For this review, take the finished solid that the model builds, in its own axes (mm). Face numbers are marked on the shaded views. A direction names the side the tool comes from. Round coordinates to 2 decimals unless told otherwise and drop trailing zeros. Loops run counter-clockwise (first coordinate to the right, second up) from the corner with the lowest first, then second, coordinate; pieces in that order, holes last.
1. To check wall thickness, follow line 1 along X through (y, z) = (-23, -36); line 2 along Y through (x, z) = (-10.5, -35); line 3 along Z through (x, y) = (-66, -9.5). State the ranges of each line that lie inside material, in increasing order.
2. Tool access review of the marked faces 5, 6 and 7: name each direction out of +Z, -Z, +X, -X, +Y, -Y from which nothing blocks a thin tool from reaching the whole face with its end or side.
3. Consider section B-B on x = 68. State the section outline as (y, z) points.
4. Clearance check with flat-ended pins moving along their axes: pin 1 Ø10 at (x, z) = (22, -87) entering from +Y; pin 2 Ø8 at (x, y) = (45, -37.5) entering from +Z; pin 3 Ø2 at (x, z) = (12, -44) entering from -Y. State where each tip first meets the part, or that it passes through.
5. Consider section D-D on x = 30. State the section outline as (y, z) points, then the cut area to 3 significant figures.
6. Consider section C-C on y = -22. State how many separate pieces and enclosed holes the cut face has, then the cut area to 3 significant figures.
7. Draft analysis for pull direction Z (two halves, no side actions). For the marked faces 1, 2, 3 and 4, state which applies: released by +Z, released by -Z, zero draft, split by the parting line, or undercut.
8. Consider section A-A on z = -50.5. State the section outline as (x, y) points, then the cut area to 3 significant figures.
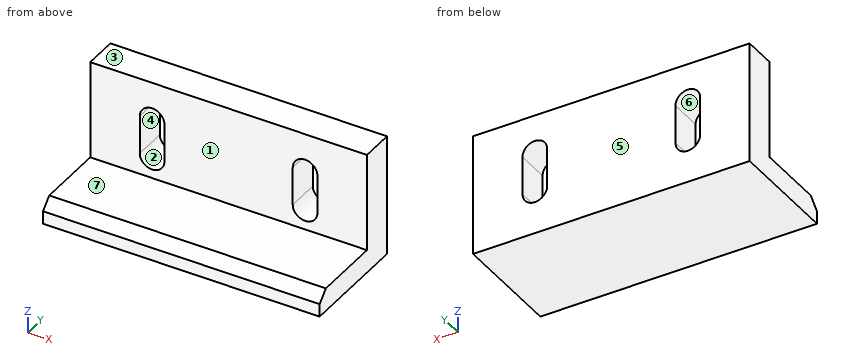
from build123d import *

# Parameters (mm, degrees)
F0_W     = 237.5140190125
F0_H     = 104.4240146875
F1_DEPTH = 28.702
F2_W     = 237.5140190125
F2_H     = 19.9324190617
F3_DEPTH = 67.564
F4_SIZE2 = 8.89
F4_SIZE  = 8.89


with BuildPart() as f1:
    # F0 (on Front) → F1 (new body)
    with BuildSketch(Plane.XZ):
        with Locations((0, -52.2120073438)):
            Rectangle(F0_W, F0_H)
        with BuildLine():
            ThreePointArc((-76.26119588, -33.1665679002), (-65.6689032912, -22.5742753114), (-55.0766107024, -33.1665679002))
            Line((-55.0766107024, -33.1665679002), (-55.0766107024, -66.2979632616))
            ThreePointArc((-55.0766107024, -66.2979632616), (-65.6689032912, -76.8902558504), (-76.26119588, -66.2979632616))
            ThreePointArc((-76.26119588, -66.2979632616), (-76.26119587, -66.2975014647), (-76.2611958398, -66.2970396679))
            Line((-76.26119588, -66.2970396679), (-76.26119588, -33.1665679002))
        make_face(mode=Mode.SUBTRACT)
        with BuildLine():
            Line((55.0766107024, -66.2979632616), (55.0766107024, -33.1665679002))
            ThreePointArc((55.0766107024, -33.1665679002), (65.6689032912, -22.5742753114), (76.26119588, -33.1665679002))
            Line((76.26119588, -33.1665679002), (76.26119588, -66.2970396679))
            Line((76.26119588, -66.2970396679), (76.26119588, -66.2979632616))
            ThreePointArc((76.26119588, -66.2979632616), (65.6689032912, -76.8902558504), (55.0766107024, -66.2979632616))
        make_face(mode=Mode.SUBTRACT)
    extrude(amount=F1_DEPTH)

    # F2 (on face) → F3 (join)
    with BuildSketch(Plane.XZ.offset(28.702)):
        with Locations((0, -94.4578051567)):
            Rectangle(F2_W, F2_H)
    extrude(amount=F3_DEPTH)

    # F4
    f4_edges = [f1.edges().sort_by_distance(p)[0] for p in [
        (0, -96.266, -84.491596),
    ]]
    chamfer(f4_edges, length=F4_SIZE, length2=F4_SIZE2)


solid = f1.part
Resolved:
1. line 1: x = -118.76 to -76.26, -55.08 to 55.08, 76.26 to 118.76
1. line 2: y = -28.7 to 0
1. line 3: z = -104.42 to -76.89, -22.58 to 0
2. face 5: +Z, -Z, +X, -X, +Y
2. face 6: +Y, -Y
2. face 7: +Z, +X, -X, -Y
3. outline: (-96.27, -104.42) - (0, -104.42) - (0, -76.63) - (-28.7, -76.63) - (-28.7, -84.49) - (-87.38, -84.49) - (-96.27, -93.38) - close; (-28.7, -22.83) - (0, -22.83) - (0, 0) - (-28.7, 0) - close
4. pin 1: stops at y = 0
4. pin 2: stops at z = -84.49
4. pin 3: stops at y = -28.7
5. outline: (-96.27, -104.42) - (0, -104.42) - (0, 0) - (-28.7, 0) - (-28.7, -84.49) - (-87.38, -84.49) - (-96.27, -93.38) - close
5. area: 4,300 mm2
6. separate pieces: 1
6. enclosed holes: 2
6. area: 22,700 mm2
7. face 1: zero draft
7. face 2: undercut
7. face 3: released by +Z
7. face 4: undercut
8. outline: (-118.76, -28.7) - (-76.26, -28.7) - (-76.26, 0) - (-118.76, 0) - close; (-55.08, -28.7) - (55.08, -28.7) - (55.08, 0) - (-55.08, 0) - close; (76.26, -28.7) - (118.76, -28.7) - (118.76, 0) - (76.26, 0) - close
8. area: 5,600 mm2
